Verification items for the finished model (mm, model axes). A direction names the side the tool comes from. Round coordinates to 2 decimals unless told otherwise and drop trailing zeros. Order: outer loops, then holes, each group sorted by start corner. A loop starts at its lowest first (then second) coordinate and runs counter-clockwise, first axis right, second up. Notation, with made-up numbers: M 11,-26.5 L 41,-26.5 A18 ccw 41,3.5 Z; hole C -34.75,27 d6. An arc over 180 degrees is marked long. Use one line per item in the form item = value. Start each with the question number.
Item 1: Cross-section at D-D on x = 5. Enter the section's corners in (y, z).
Item 2: Thickness scan on probe 1 along Z at (x, y) = (7, 3.5); probe 2 along X at (y, z) = (-0.5, -0.5); probe 3 along X at (y, z) = (5.5, -2). Record the ranges inside material, lowest first. Write a range as [from, to].
Item 3: Cross-section at B-B on z = -0.25. Enter the section's corners in (x, y).
Item 4: Release check for a two-part mould opening along Y. For faces 1 (the cylindrical face through (6.28, 5.47, -1.43)), 2 (the flat face through (3, 3, 0.1)), 3 (the cylindrical face through (8.389, -2.408, 4.967)), 4 (the cylindrical face through (8.408, 8.389, 4.967)) record: +Y half, -Y half, draft (parallel to the pull), parting line (faces both ways), or undercut.
Item 5: Tool access check on faces 5 (the flat face through (3, 3, 9.7)), 6 (the cylindrical face through (0.323, 0.506, -1.428)). Record the directions out of +Z, -Z, +X, -X, +Y, -Y that give a thin tool (end or side, any length) a straight path to the whole face; none if there is none.
Item 6: Cross-section at A-A on y = 6. Enter the section's corners in (x, z).
Item 7: Cross-section at C-C on x = 0. Enter the section's corners in (y, z), then the cut area to 3 significant figures.
from build123d import *

# Parameters (mm, degrees)
SKETCH001_R  = 0.6
PAD001_DEPTH = 3.5
SKETCH_W     = 11.5
SKETCH_H     = 11.5
PAD_DEPTH    = 9.6
FILLET_R     = 1.2


with BuildPart() as pad001:
    # Sketch001 → Pad001 (new body)
    with BuildSketch(Plane.XY.offset(0.5)):
        Circle(SKETCH001_R)
        with Locations((6, 6)):
            Circle(SKETCH001_R)
    extrude(amount=-PAD001_DEPTH)


with BuildPart() as obj1:
    # Sketch → Pad (new body)
    with BuildSketch(Plane.XY.offset(0.1)):
        with Locations((3, 3)):
            Rectangle(SKETCH_W, SKETCH_H)
    extrude(amount=PAD_DEPTH)

    # Fillet
    fillet_edges = [obj1.edges().sort_by_distance(p)[0] for p in [
        (8.75, -2.75, 4.9),
        (8.75, 8.75, 4.9),
        (-2.75, -2.75, 4.9),
        (-2.75, 8.75, 4.9),
    ]]
    fillet(fillet_edges, radius=FILLET_R)

    # obj1: union Pad001
    add(pad001.part)


solid = obj1.part
Output values:
q1.outline = M -2.75,0.1 L 8.75,0.1 L 8.75,9.7 L -2.75,9.7 Z
q2.probe_1 = [0.1, 9.7]
q2.probe_2 = [-0.33, 0.33]
q2.probe_3 = [5.67, 6.33]
q3.outline = C 0,0 d1.2; C 6,6 d1.2
q4.face_1 = parting line
q4.face_2 = draft
q4.face_3 = -Y half
q4.face_4 = +Y half
q5.face_5 = +Z, +X, -X, +Y, -Y
q5.face_6 = -Z
q6.outline = M -2.75,0.1 L 5.4,0.1 L 5.4,-3 L 6.6,-3 L 6.6,0.1 L 8.75,0.1 L 8.75,9.7 L -2.75,9.7 Z
q7.outline = M -2.75,0.1 L -0.6,0.1 L -0.6,-3 L 0.6,-3 L 0.6,0.1 L 8.75,0.1 L 8.75,9.7 L -2.75,9.7 Z
q7.area = 114 mm2
